from build123d import *

# Parameters (mm, degrees)
F0_R     = 63.5
F0_R_2   = 10
F1_DEPTH = 10


with BuildPart() as f1:
    # F0 (on Top) → F1 (new body)
    with BuildSketch(Plane.XY):
        Circle(F0_R)
        with BuildLine():
            ThreePointArc((1.548061, 15.4225), (10.960155, 10.960155), (15.4225, 1.548061))
            ThreePointArc((15.4225, 1.548061), (16.568264, 1.123082), (17.05, 0))
            ThreePointArc((17.05, 0), (16.568264, -1.123082), (15.4225, -1.548061))
            ThreePointArc((15.4225, -1.548061), (10.960155, -10.960155), (1.548061, -15.4225))
            ThreePointArc((1.548061, -15.4225), (1.549515, -15.461238), (1.55, -15.5))
            ThreePointArc((1.55, -15.5), (-0.038762, -17.049515), (-1.548061, -15.4225))
            ThreePointArc((-1.548061, -15.4225), (-10.960155, -10.960155), (-15.4225, -1.548061))
            ThreePointArc((-15.4225, -1.548061), (-17.05, 0), (-15.4225, 1.548061))
            ThreePointArc((-15.4225, 1.548061), (-10.960155, 10.960155), (-1.548061, 15.4225))
            ThreePointArc((-1.548061, 15.4225), (-0.038762, 17.049515), (1.55, 15.5))
            ThreePointArc((1.55, 15.5), (1.549515, 15.461238), (1.548061, 15.4225))
        make_face(mode=Mode.SUBTRACT)
        with BuildLine():
            ThreePointArc((15.4225, -1.548061), (13.95, 0), (15.4225, 1.548061))
            ThreePointArc((15.4225, 1.548061), (10.960155, 10.960155), (1.548061, 15.4225))
            ThreePointArc((1.548061, 15.4225), (0, 13.95), (-1.548061, 15.4225))
            ThreePointArc((-1.548061, 15.4225), (-10.960155, 10.960155), (-15.4225, 1.548061))
            ThreePointArc((-15.4225, 1.548061), (-14.376918, 1.068264), (-13.95, 0))
            ThreePointArc((-13.95, 0), (-14.376918, -1.068264), (-15.4225, -1.548061))
            ThreePointArc((-15.4225, -1.548061), (-10.960155, -10.960155), (-1.548061, -15.4225))
            ThreePointArc((-1.548061, -15.4225), (0, -13.95), (1.548061, -15.4225))
            ThreePointArc((1.548061, -15.4225), (10.960155, -10.960155), (15.4225, -1.548061))
        make_face()
        Circle(F0_R_2, mode=Mode.SUBTRACT)
    extrude(amount=F1_DEPTH)


solid = f1.part
Here's how the part is built. I have some questions about the finished solid (model axes, mm). Round coordinates to 2 decimals unless told otherwise and drop trailing zeros. Loops run counter-clockwise (first coordinate to the right, second up) from the corner with the lowest first, then second, coordinate; pieces in that order, holes last.
1. If we section it at B-B on x = 0: Write out the boundary of the cut face in (y, z), plus the area to 3 significant figures.
Answer list:
outline: (-63.5, 0) - (-17.05, 0) - (-17.05, 10) - (-63.5, 10) - close; (-13.95, 0) - (-10, 0) - (-10, 10) - (-13.95, 10) - close; (10, 0) - (13.95, 0) - (13.95, 10) - (10, 10) - close; (17.05, 0) - (63.5, 0) - (63.5, 10) - (17.05, 10) - close
area: 1,010 mm2
2. If we section it at A-A on z = 6.5: Write out the boundary of the cut face in (x, y).
Answer list:
outline: circle Ø127 at (0, 0); hole (-15.42, -1.55) arc R1.55 ccw to (-13.95, 0) arc R1.55 ccw to (-15.42, 1.55) arc R1.55 ccw (long way) to start; hole circle Ø20 at (0, 0); hole (1.55, -15.5) arc R1.55 ccw to (1.55, -15.42) arc R1.55 ccw (long way) to start; hole (1.55, 15.42) arc R1.55 ccw to (1.55, 15.5) arc R1.55 ccw (long way) to start; hole (15.42, -1.55) arc R1.55 ccw to (17.05, 0) arc R1.55 ccw to (15.42, 1.55) arc R1.55 ccw to start
3. For P1, Ø5, axis at x = -20.5, y = 43.5, coming from the -Z side; P2, Ø1, axis at y = -13, z = 5.5, coming from the -X side; P3, Ø6, axis at y = 39.5, z = 1, coming from the +X side; P4, Ø2, axis at y = -45.5, z = 6.5, coming from the +X side, each with a flat end and sliding along its axis, tell me the tip position at first contact or that it passes through.
Answer list:
P1: stops at z = 0
P2: stops at x = -62.26
P3: stops at x = 51.96
P4: stops at x = 45.3
4. We'd pull the mould along X, two halves only. Please class faces 1 (the face through (-13.77, -61.99, 4.93)), 2 (the face through (-2.17, -9.76, 4.93)), 3 (the face through (13, 1, 10)): +X half, -X half, draft (parallel to the pull), parting line (faces both ways), or undercut.
Answer list:
face 1: parting line
face 2: undercut
face 3: draft
5. If I drill on line 1 along Y through (x, z) = (14.5, 1.25); line 2 along X through (y, z) = (-8, 1.25); line 3 along Y through (x, z) = (-17.5, 3.25), over which ranges is the centre line in solid material (lowest first)?
Answer list:
line 1: y = -61.82 to -1.18, 1.18 to 61.82
line 2: x = -62.99 to -6, 6 to 62.99
line 3: y = -61.04 to 61.04
6. If we section it at C-C on y = 28.5: Write out the boundary of the cut face in (x, z), plus the area to 3 significant figures.
Answer list:
outline: (-56.75, 0) - (56.75, 0) - (56.75, 10) - (-56.75, 10) - close
area: 1,130 mm2
